Geometry check sheet. Reference: drawing and pictorial views, mm from the part's lowest x, y, z. A direction names the side the tool comes from. Give positions to 0.01 mm unless a question says otherwise; leave off trailing zeros. Write each loop counter-clockwise with the first axis right and the second up, starting at its lowest first coordinate (ties: lowest second). Pieces come first, ordered by that corner, then holes. Notation, with made-up numbers: (74.25, 61) -> (82.25, 61) arc R35 cw to (82.25, 97) -> close; hole circle Ø6 at (39, -35). An arc over 180 degrees is marked (long way). Return JSON: item names as keys, results as strings.
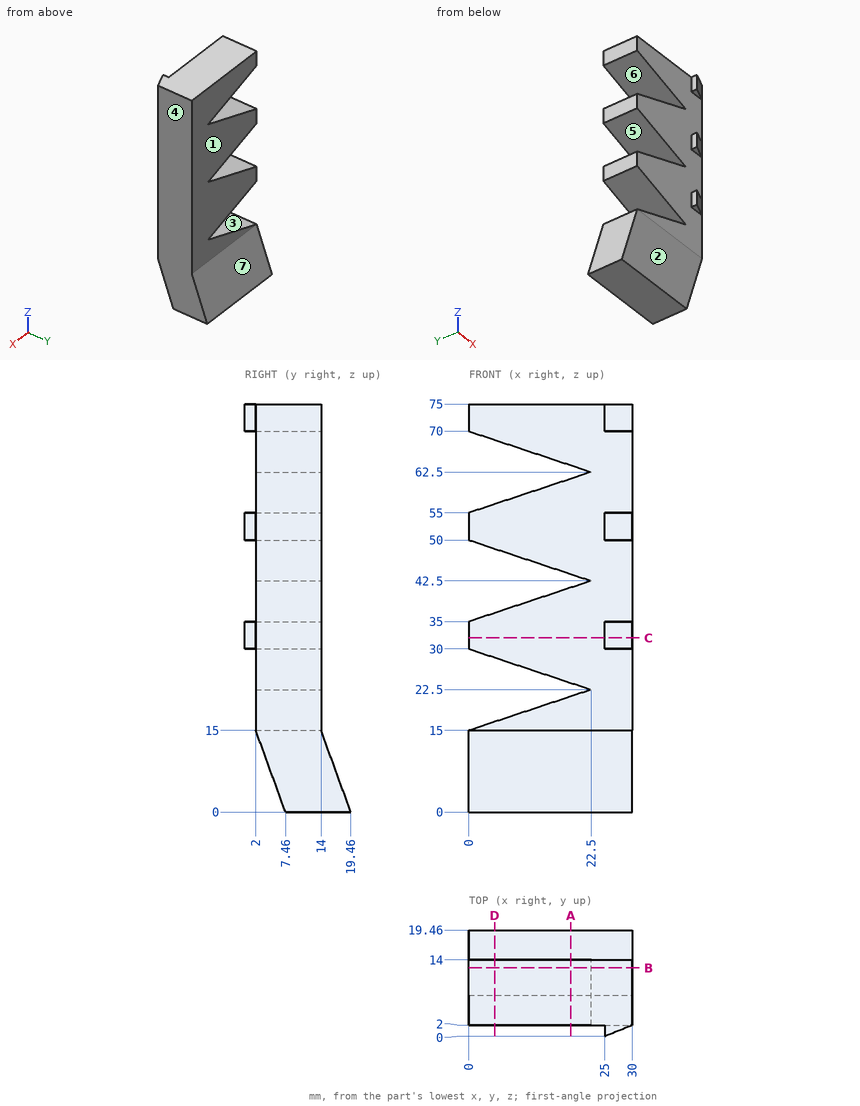
(1) Cross-section at A-A on x = 18.75. Enter the section's corners in (y, z).
Reply:
{"outline": "(2, 15) -> (7.46, 0) -> (19.46, 0) -> (14, 15) -> (14, 21.25) -> (2, 21.25) -> close; (2, 23.75) -> (14, 23.75) -> (14, 41.25) -> (2, 41.25) -> close; (2, 43.75) -> (14, 43.75) -> (14, 61.25) -> (2, 61.25) -> close; (2, 63.75) -> (14, 63.75) -> (14, 75) -> (2, 75) -> close"}
(2) Release check for a two-part mould opening along Z. For the marked faces 4, 5, 6 and 7 record: pulls with the +Z half, pulls with the -Z half, needs draft (parallel to the pull), parting line crosses it, or undercut.
Reply:
{"face 4": "needs draft", "face 5": "undercut", "face 6": "undercut", "face 7": "pulls with the +Z half"}
(3) Set-up check for the marked faces 1, 2 and 3: record each of +Z, -Z, +X, -X, +Y, -Y from which the full face is reachable in a straight line by a thin tool's end or side.
Reply:
{"face 1": "+Z, +X, -X, +Y", "face 2": "-Z, +X, -X, -Y", "face 3": "-X, +Y, -Y"}
(4) Cross-section at B-B on y = 12.5. Enter the section's corners in (x, z).
Reply:
{"outline": "(0, 0) -> (30, 0) -> (30, 75) -> (0, 75) -> (0, 70) -> (22.5, 62.5) -> (0, 55) -> (0, 50) -> (22.5, 42.5) -> (0, 35) -> (0, 30) -> (22.5, 22.5) -> (0, 15) -> close"}
(5) Cross-section at D-D on x = 4.75. Enter the section's corners in (y, z), then the cut area to 3 significant figures.
Reply:
{"outline": "(2, 15) -> (7.46, 0) -> (19.46, 0) -> (14, 15) -> (14, 16.58) -> (2, 16.58) -> close; (2, 28.42) -> (14, 28.42) -> (14, 36.58) -> (2, 36.58) -> close; (2, 48.42) -> (14, 48.42) -> (14, 56.58) -> (2, 56.58) -> close; (2, 68.42) -> (14, 68.42) -> (14, 75) -> (2, 75) -> close", "area": "474 mm^2"}
(6) Thickness scan on L1, parallel to Z at x = 19, y = 9.5; L2, parallel to Z at x = 13.5, y = 7.75; L3, parallel to Y at x = 2.5, z = 52. Record the ranges inside material, lowest first.
Reply:
{"L1": "0 to 21.33, 23.67 to 41.33, 43.67 to 61.33, 63.67 to 75", "L2": "0 to 19.5, 25.5 to 39.5, 45.5 to 59.5, 65.5 to 75", "L3": "2 to 14"}
(7) Depth check by flat-ended pin: pin 1 Ø12 at (x, z) = (10, 60.5) entering from -Y; pin 2 Ø5 at (y, z) = (4.5, 52.5) entering from -X; pin 3 Ø0.6 at (x, y) = (27.5, 1) entering from -Z; pin 4 Ø0.6 at (y, z) = (1, 32) entering from -X. Enter the tip coordinate at first touch or a pass-through.
Reply:
{"pin 1": "y = 2", "pin 2": "x = 0", "pin 3": "z = 30", "pin 4": "x = 25"}
(8) Cross-section at C-C on z = 32. Enter the section's corners in (x, y), then the cut area to 3 significant figures.
Reply:
{"outline": "(0, 2) -> (25, 2) -> (25, 0) -> (30, 2) -> (30, 14) -> (0, 14) -> close", "area": "365 mm^2"}
